```python
from build123d import *

# Parameters (mm, degrees)
F0_W      = 25
F0_H      = 30
F0_W_2    = 23.2
F0_H_2    = 28.2
F1_DEPTH  = 50
F2_W      = 25
F2_H      = 30
F3_DEPTH  = 1
F4_W      = 1
F4_H      = 1
F5_DEPTH  = 1
F6_W      = 22
F6_H      = 6
F7_DEPTH  = 10
F8_R      = 1.5
F9_DEPTH  = 5
F11_DEPTH = 0.1


with BuildPart() as f1:
    # F0 (on Top) → F1 (new body)
    with BuildSketch(Plane.XY):
        Rectangle(F0_W, F0_H)
        Rectangle(F0_W_2, F0_H_2, mode=Mode.SUBTRACT)
    extrude(amount=F1_DEPTH)

    # F2 (on face) → F3 (join)
    with BuildSketch(Plane.XY.offset(50)):
        Rectangle(F2_W, F2_H)
    extrude(amount=-F3_DEPTH)

    # F4 (on face) → F5 (join)
    with BuildSketch(Plane.YZ.offset(12.5)):
        with Locations((-9.5, 20.5)):
            Rectangle(F4_W, F4_H)
    extrude(amount=F5_DEPTH)

    # F6 (on face) → F7 (cut)
    with BuildSketch(Plane.XZ.offset(15)):
        with Locations((0, 3)):
            Rectangle(F6_W, F6_H)
    extrude(amount=-F7_DEPTH, mode=Mode.SUBTRACT)

    # F8 (on face) → F9 (cut)
    with BuildSketch(Plane(origin=(0, 15, 0), x_dir=(-1, 0, 0), z_dir=(0, 1, 0))):
        Circle(F8_R)
    extrude(amount=-F9_DEPTH, mode=Mode.SUBTRACT)

    # F10 (on face) → F11 (cut)
    with BuildSketch(Plane.YZ.offset(12.5)):
        Polygon((14.5, 0.6), (-14.5, 0.6), (-14.5, 50), (-15, 50), (-15, 0), (15, 0), (15, 50), (14.5, 50), align=None)
    extrude(amount=-F11_DEPTH, mode=Mode.SUBTRACT)


solid = f1.part
```
Could you check a few things on this model? Use its own coordinates, in mm. A direction names the side the tool comes from. Coordinates: 2 decimals unless noted, no trailing zeros. Order: outer loops, then holes, each group sorted by start corner. A loop starts at its lowest first (then second) coordinate and runs counter-clockwise, first axis right, second up. Notation, with made-up numbers: M 0,-3.5 L 14,-3.5 A29 ccw 14,30.5 Z; hole C -18,85 d10. An arc over 180 degrees is marked long. Use one line per item in the form item = value. Start each with the question number.
1. Suppose I cut it at C-C on y = -5. Write out the boundary of the cut face in (x, z), then the cut area to 3 significant figures.
2. For pin 1 (1 mm diameter, centred on y = 9, z = 15, fed in from +X); pin 2 (0.5 mm diameter, centred on x = 13, y = -9.5, fed in from +Z); pin 3 (1.1 mm diameter, centred on x = 13, z = 20.5, fed in from +Y), each with a flat end and sliding along its axis, tell me the tip position at first contact or that it passes through.
3. Please list where these lines run through material, in increasing order: line 1 (Y direction, x = 7.5, z = 7); line 2 (X direction, y = 1, z = 40.5); line 3 (Z direction, x = -7.75, y = 9.75).
4. Suppose I cut it at D-D on x = 0. Write out the boundary of the cut face in (y, z).
5. Suppose I cut it at B-B on x = 8.5. Write out the boundary of the cut face in (y, z).
6. On a 3-axis mill with a long thin cutter (end or side, diameter ignored), from which of +Z, -Z, +X, -X, +Y, -Y can I reach the whole of each face in a straight line? I mean faces 1 (the flat face through (11.6, 0, 24)), 2 (the flat face through (13, -10, 20.5)), 3 (the flat face through (13, -9.5, 20)). Say none if no direction works.
7. Suppose I cut it at A-A on z = 39.5. Write out the boundary of the cut face in (x, y), then the cut area to 3 significant figures.
8. We'd pull the mould along Y, two halves only. Please class faces 4 (the flat face through (0, -15, 25)), 5 (the flat face through (0, 15, 25)), 6 (the flat face through (0, -14.1, 24)), 7 (the flat face through (13, -9.5, 21)): +Y half, -Y half, draft (parallel to the pull), parting line (faces both ways), or undercut.
Geometry says:
q1.outline = M -12.5,0 L -11.6,0 L -11.6,49 L 11.6,49 L 11.6,0 L 12.4,0 L 12.4,0.6 L 12.5,0.6 L 12.5,50 L -12.5,50 Z
q1.area = 113 mm^2
q2.pin_1 = 12.5
q2.pin_2 = 21
q2.pin_3 = 14.5
q3.line_1 = -15 to -14.1, 14.1 to 15
q3.line_2 = -12.5 to -11.6, 11.6 to 12.5
q3.line_3 = 49 to 50
q4.outline = M -15,6 L -14.1,6 L -14.1,49 L 14.1,49 L 14.1,1.5 L 15,1.5 L 15,50 L -15,50 Z
q5.outline = M -15,6 L -14.1,6 L -14.1,49 L 14.1,49 L 14.1,0 L 15,0 L 15,50 L -15,50 Z
q6.face_1 = -Z
q6.face_2 = +Z, -Z, +X, -Y
q6.face_3 = -Z, +X, +Y, -Y
q7.outline = M -12.5,-15 L 12.4,-15 L 12.4,-14.5 L 12.5,-14.5 L 12.5,14.5 L 12.4,14.5 L 12.4,15 L -12.5,15 Z; hole M -11.6,-14.1 L 11.6,-14.1 L 11.6,14.1 L -11.6,14.1 Z
q7.area = 95.7 mm^2
q8.face_4 = -Y half
q8.face_5 = +Y half
q8.face_6 = undercut
q8.face_7 = draft
